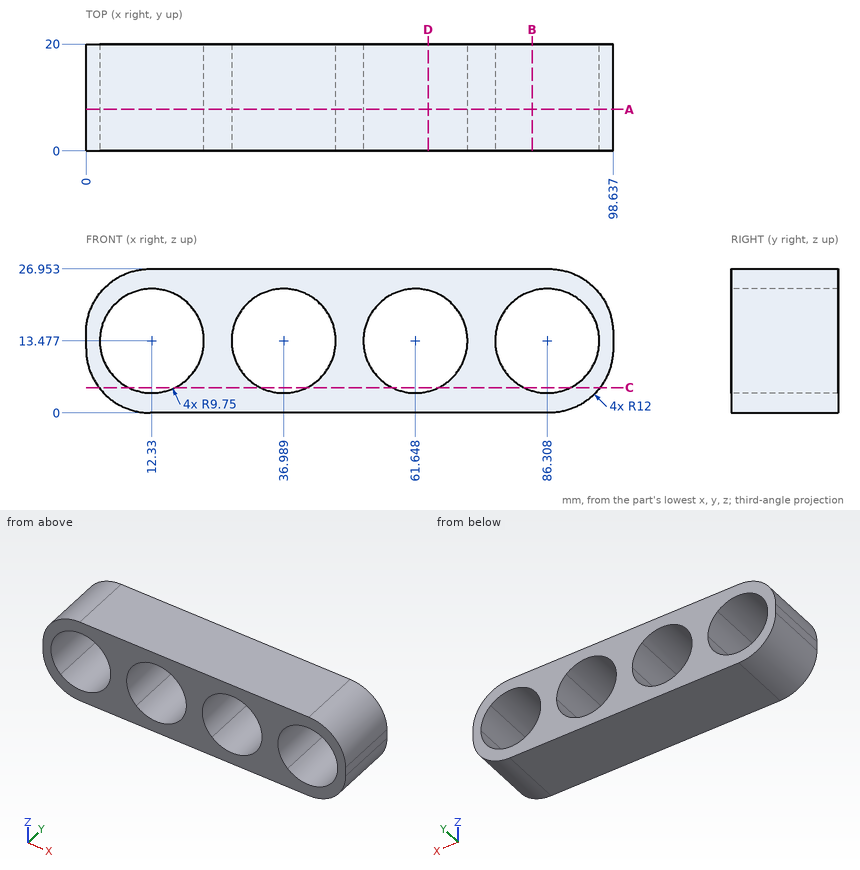
Could you check a few things on this drawing? It's one solid part, dimensions in mm from its lowest x, y, z. Give positions to 0.01 mm unless a question says otherwise; leave off trailing zeros. Write each loop counter-clockwise with the first axis right and the second up, starting at its lowest first coordinate (ties: lowest second). Pieces come first, ordered by that corner, then holes.
(1) Will these pins go through, and if not, where does the flat tip stop? pin 1 (8 mm diameter, centred on y = 13.5, z = 17.5, fed in from +X); pin 2 (10 mm diameter, centred on x = 13, z = 12.5, fed in from -Y).
Output values:
pin 1: stops at x = 98.64
pin 2: passes through
(2) If I drill on L1, parallel to X at y = 14.5, z = 14 (1 decimal); L2, parallel to Z at x = 62, y = 12; L3, parallel to X at y = 6.25, z = 15.75, over which ranges is the centre line in solid material (lowest first)?
Output values:
L1: x = 0 to 2.6, 22.1 to 27.3, 46.7 to 51.9, 71.4 to 76.6, 96 to 98.6
L2: z = 0 to 3.73, 23.22 to 26.95
L3: x = 0.03 to 2.85, 21.81 to 27.51, 46.47 to 52.17, 71.13 to 76.83, 95.79 to 98.61
(3) Imagine slicing it at B-B, the plane x = 83.5. Write out the boundary of the cut face in (y, z), and give its area (3 significant figures).
Output values:
outline: (0, 0) - (20, 0) - (20, 4.14) - (0, 4.14) - close; (0, 22.81) - (20, 22.81) - (20, 26.95) - (0, 26.95) - close
area: 166 mm2
(4) Imagine slicing it at A-A, the plane y = 7.75. Write out the boundary of the cut face in (x, z), and give its area (3 significant figures).
Output values:
outline: (0, 12) arc R12 ccw to (12, 0) - (86.64, 0) arc R12 ccw to (98.64, 12) - (98.64, 14.95) arc R12 ccw to (86.64, 26.95) - (12, 26.95) arc R12 ccw to (0, 14.95) - close; hole circle Ø19.5 at (12.33, 13.48); hole circle Ø19.5 at (36.99, 13.48); hole circle Ø19.5 at (61.65, 13.48); hole circle Ø19.5 at (86.31, 13.48)
area: 1,340 mm2
(5) Imagine slicing it at C-C, the plane z = 4.75. Write out the boundary of the cut face in (x, y), and give its area (3 significant figures).
Output values:
outline: (2.44, 0) - (7.98, 0) - (7.98, 20) - (2.44, 20) - close; (16.68, 0) - (32.64, 0) - (32.64, 20) - (16.68, 20) - close; (41.34, 0) - (57.3, 0) - (57.3, 20) - (41.34, 20) - close; (66, 0) - (81.96, 0) - (81.96, 20) - (66, 20) - close; (90.66, 0) - (96.2, 0) - (96.2, 20) - (90.66, 20) - close
area: 1,180 mm2
(6) Imagine slicing it at D-D, the plane x = 64. Write out the boundary of the cut face in (y, z) (1 decimal), and give its area (3 significant figures).
Output values:
outline: (0, 0) - (20, 0) - (20, 4) - (0, 4) - close; (0, 22.9) - (20, 22.9) - (20, 27) - (0, 27) - close
area: 161 mm2
